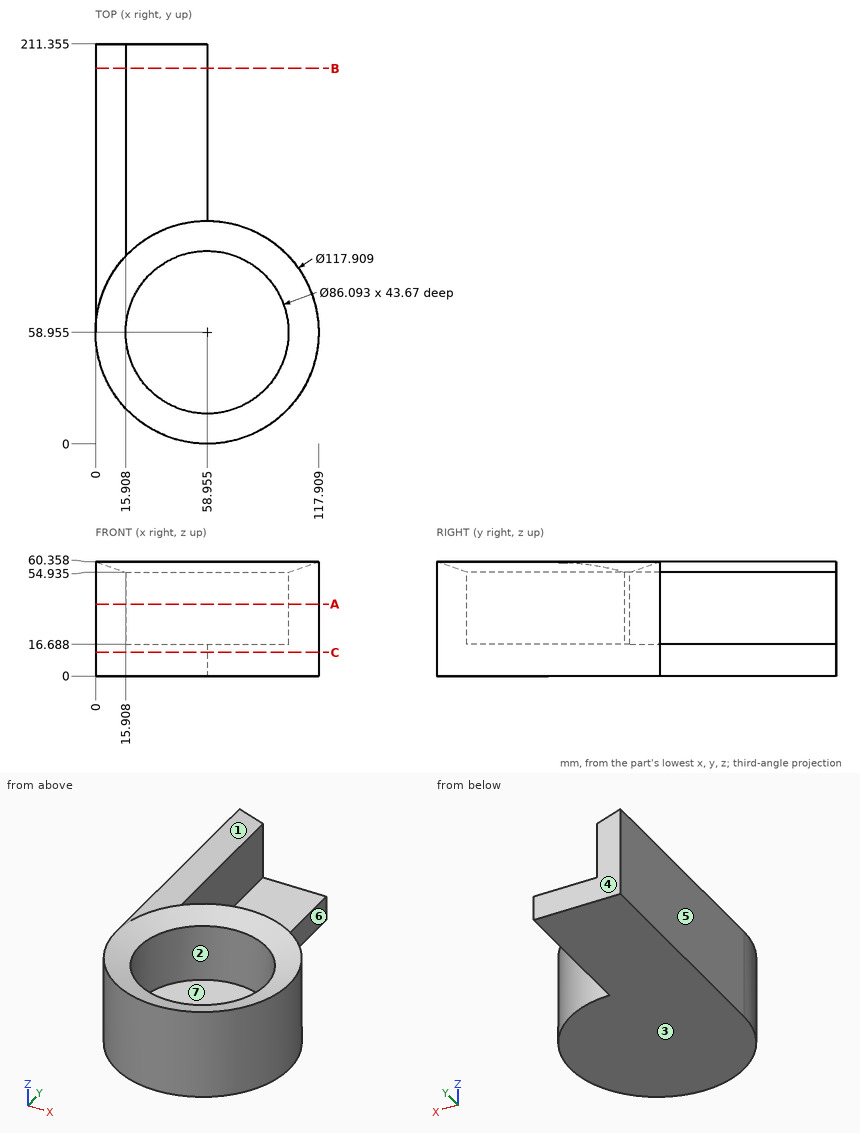
Could you check a few things on this drawing? It's one solid part, dimensions in mm from its lowest x, y, z. A direction names the side the tool comes from. Round coordinates to 2 decimals unless told otherwise and drop trailing zeros. Order: outer loops, then holes, each group sorted by start corner. A loop starts at its lowest first (then second) coordinate and runs counter-clockwise, first axis right, second up. Notation, with made-up numbers: (82, -34) -> (102, -34) arc R36 cw to (102, 3) -> close; hole circle Ø7 at (-28, 71). An arc over 180 degrees is marked (long way). One line per question, with ' | ' between items.
Q1. We'd pull the mould along X, two halves only. Please class the marked faces 4, 5, 6 and 7: released by +X, released by -X, zero draft, split by the parting line, or undercut.
Computed values:
face 4: zero draft | face 5: released by -X | face 6: released by +X | face 7: undercut
Q2. Which directions (+Z, -Z, +X, -X, +Y, -Y) give clear straight access to the entire face, cutting with the end or side of a thin tool? Please do the marked faces 1, 2 and 3.
Computed values:
face 1: +Z, +Y | face 2: +Z | face 3: -Z, +X, -X, +Y, -Y
Q3. I'm going to push flat-ended pins straight in: pin 1 (3 mm diameter, centred on y = 92.5, z = 42.5, fed in from +X); pin 2 (5 mm diameter, centred on x = 83, z = 26, fed in from -Y); pin 3 (8 mm diameter, centred on x = 76, z = 42, fed in from -Y). Where does each tip first touch, or does it pass through?
Computed values:
pin 1: x = 108.44 | pin 2: y = 4.08 | pin 3: y = 1.46
Q4. If we section it at B-B on y = 198.5: Write out the boundary of the cut face in (x, z) (1 decimal).
Computed values:
outline: (0, 0) -> (59, 0) -> (59, 16.7) -> (15.9, 16.7) -> (15.9, 54.9) -> (0, 60.4) -> close
Q5. If we section it at A-A on z = 38: Write out the boundary of the cut face in (x, y) (1 decimal), plus the area to 3 significant figures.
Computed values:
outline: (0, 59) arc R59 ccw (long way) to (15.9, 99.2) -> (15.9, 211.4) -> (0, 211.4) -> close; hole circle Ø86.1 at (59, 59) | area: 7,080 mm²
Q6. If we section it at C-C on z = 12.5: Write out the boundary of the cut face in (x, y) (1 decimal).
Computed values:
outline: (0, 59) arc R59 ccw (long way) to (59, 117.9) -> (59, 211.4) -> (0, 211.4) -> close
Q7. If I drill on line 1 (Z direction, x = 29, y = 200.5); line 2 (Y direction, x = 49, z = 32) (1 decimal); line 3 (X direction, y = 168.5, z = 13) (1 decimal), over which ranges is the centre line in solid material (lowest first)? Write a range as from..to.
Computed values:
line 1: 0..16.69 | line 2: 0.8..17.1, 100.8..117.1 | line 3: 0..59
